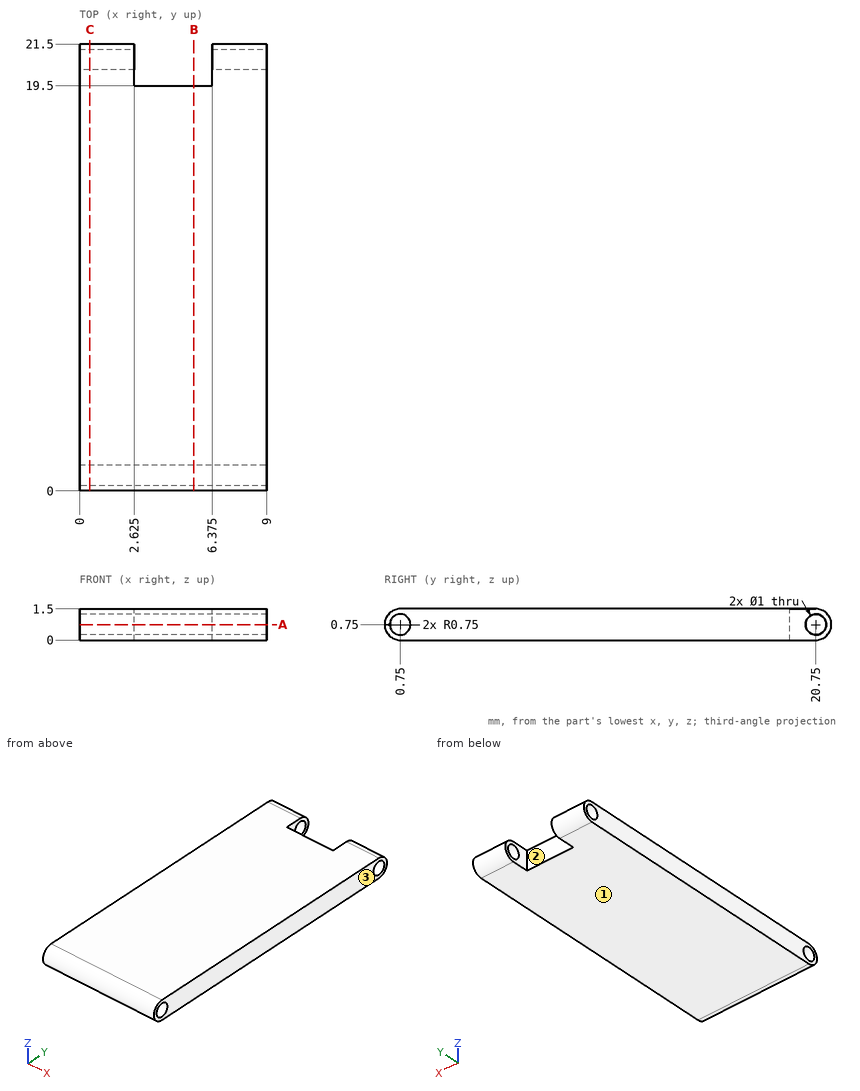
Print and shaded views of the part. All mm, measured from the part's lowest x, y and z. Coordinates: 2 decimals unless noted, no trailing zeros. Order: outer loops, then holes, each group sorted by start corner. A loop starts at its lowest first (then second) coordinate and runs counter-clockwise, first axis right, second up. Notation, with made-up numbers: M -39,87 L -32,87 A12 ccw -32,106 Z; hole C 14,41.25 d8. An arc over 180 degrees is marked long. Write each question's results on one line, items separated by ' | '. Start each with the question number.
Q1. Cut at C-C (x = 0.5). List the corners of the cut face in (y, z), then the cut area to 3 significant figures.
Q2. Cut at B-B (x = 5.5). List the corners of the cut face in (y, z).
Q3. Drill centre lines: probe 1 along Y at (x, z) = (8, 0.7); probe 2 along Z at (x, y) = (7.6, 20.75); probe 3 along X at (y, z) = (20, 0.9) (3 decimals). Where is each one in solid material? Low to high. Write a range as from..to.
Q4. Pull direction X, two halves, no side cores. Call the marked faces 1, 2 and 3: +X half, -X half, draft (parallel to the pull), parting line (faces both ways), or undercut.
Q5. Flat gauge pin, fed straight in: P1, Ø0.8, axis at x = 4.5, z = 0.5, coming from the +Y side. Where does the tip first touch, or does it go through?
Q6. Cut at A-A (z = 0.75). List the corners of the cut face in (x, y) (3 decimals).
Found:
1) outline: M 0.75,0 L 20.75,0 A0.75 ccw 20.75,1.5 L 0.75,1.5 A0.75 ccw Z; hole C 0.75,0.75 d1; hole C 20.75,0.75 d1 | area: 30.2 mm²
2) outline: M 0.75,0 L 19.5,0 L 19.5,1.5 L 0.75,1.5 A0.75 ccw Z; hole C 0.75,0.75 d1
3) probe 1: 0..0.25, 1.25..20.25, 21.25..21.5 | probe 2: 0..0.25, 1.25..1.5 | probe 3: 0..2.625, 6.375..9
4) face 1: draft | face 2: undercut | face 3: +X half
5) P1: y = 19.5
6) outline: M 0,0 L 9,0 L 9,0.25 L 0,0.25 Z; M 0,1.25 L 9,1.25 L 9,20.25 L 6.375,20.25 L 6.375,19.5 L 2.625,19.5 L 2.625,20.25 L 0,20.25 Z; M 0,21.25 L 2.625,21.25 L 2.625,21.5 L 0,21.5 Z; M 6.375,21.25 L 9,21.25 L 9,21.5 L 6.375,21.5 Z
